from build123d import *

# Parameters (mm, degrees)
PAD004_DEPTH         = 30
SKETCH011_R          = 20.5
POCKET004_DEPTH      = 42.931486
POCKET004_DEPTH_BACK = 27.070514
POCKET005_DEPTH      = 263.838706
POCKET005_DEPTH_BACK = 247.977735
SKETCH013_R          = 2.7
POCKET006_DEPTH      = 220.90822
POCKET006_DEPTH_BACK = 250.90822
POCKET007_DEPTH      = 244.092718
SKETCH024_W          = 115.08152
SKETCH024_H          = 98.641312
POCKET017_DEPTH      = 2


with BuildPart() as part:
    # Sketch010 → Pad004 (new body)
    with BuildSketch(Plane.XZ):
        Polygon((-27.069514, 0), (-17.069514, 40), (32.930486, 40), (42.930486, 0), (32.930486, -40), (-17.069514, -40), align=None)
    extrude(amount=PAD004_DEPTH)

    # Sketch011 → Pocket004 (cut, two sides)
    with BuildSketch(Plane.YZ) as pocket004_sk:
        Circle(SKETCH011_R)
    extrude(amount=POCKET004_DEPTH, mode=Mode.SUBTRACT)
    extrude(pocket004_sk.sketch, amount=-POCKET004_DEPTH_BACK, mode=Mode.SUBTRACT)

    # Sketch012 → Pocket005 (cut, two sides)
    with BuildSketch(Plane.YZ) as pocket005_sk:
        Polygon((-36.13987, 42.447654), (-6.815503, 42.447654), (-6.815503, 35.734174), (-23.345354, 26.19066), (-36.13987, 13.396144), align=None)
    pocket005 = extrude(amount=POCKET005_DEPTH, mode=Mode.SUBTRACT) + extrude(pocket005_sk.sketch, amount=-POCKET005_DEPTH_BACK, mode=Mode.SUBTRACT)

    # Mirrored001: Pocket005 across Sketch012 H_Axis
    add(pocket005.mirror(Plane.XY), mode=Mode.SUBTRACT)

    # Sketch013 → Pocket006 (cut, two sides)
    with BuildSketch(Plane.XZ) as pocket006_sk:
        with Locations((-7.069514, 30)):
            Circle(SKETCH013_R)
        with Locations((22.930486, 30)):
            Circle(SKETCH013_R)
    pocket006 = extrude(amount=-POCKET006_DEPTH, mode=Mode.SUBTRACT) + extrude(pocket006_sk.sketch, amount=POCKET006_DEPTH_BACK, mode=Mode.SUBTRACT)

    # Mirrored002: Pocket006 across Sketch013 H_Axis
    add(pocket006.mirror(Plane(origin=(0, 0, 0), x_dir=(0, -1, 0), z_dir=(0, 0, 1))), mode=Mode.SUBTRACT)

    # Sketch014 (on Face5 of Mirrored002) → Pocket007 (cut, through all)
    with BuildSketch(Plane.XZ.offset(6.815503)):
        Polygon((-11.874352, 24.888732), (27.735323, 24.888732), (33.996942, 35.734174), (-18.135971, 35.734174), align=None)
    pocket007 = extrude(amount=POCKET007_DEPTH, mode=Mode.SUBTRACT)

    # Mirrored003: Pocket007 across Sketch014 H_Axis
    add(pocket007.mirror(Plane(origin=(0, -6.815503, 0), x_dir=(0, -1, 0), z_dir=(0, 0, 1))), mode=Mode.SUBTRACT)

    # Sketch024 (on Face12 of Mirrored003) → Pocket017 (cut)
    with BuildSketch(Plane(origin=(0, 0, 0), x_dir=(1, 0, 0), z_dir=(0, 1, 0))):
        with Locations((8.455631, -2.089874)):
            Rectangle(SKETCH024_W, SKETCH024_H)
    extrude(amount=-POCKET017_DEPTH, mode=Mode.SUBTRACT)


with BuildPart() as part_1:
    # Body003 placement: moved
    add(part.part.moved(Location((0, -40, 0))))


solid = part_1.part
Source: CAD feature listing. Evaluate the final solid. Frame: model axes, mm. A direction names the side the tool comes from. Give positions to 0.01 mm unless a question says otherwise; leave off trailing zeros. Loops run counter-clockwise (first coordinate to the right, second up) from the corner with the lowest first, then second, coordinate; pieces in that order, holes last. Notation, with made-up numbers: (-4, -31) -> (40, -31) arc R32 ccw to (40, -5) -> close; hole circle Ø11 at (9.5, 4). An arc over 180 degrees is marked (long way). Use a Markdown table: item, result. Add a question column.
1) Section query C-C, the plane x = -8.5. Return the cut outline in (y, z), then the cut area to 3 significant figures.
2) Line query: line 1 along Z through (x, y) = (-0.5, -44); line 2 along Z through (x, y) = (32, -50); line 3 along Z through (x, y) = (13.5, -61.5). Output: solid intervals per line, ascending. Write a range as [from, to].
3) Section query D-D, the plane x = 2. Return the cut outline in (y, z), then the cut area to 3 significant figures.
4) Section query A-A, the plane z = 31. Return the cut outline in (x, y).
5) First-contact query: pin 1 (5 mm diameter, centred on y = -67, z = -5, fed in from -X); pin 2 (8 mm diameter, centred on x = 4.5, z = -1, fed in from +Y); pin 3 (7.5 mm diameter, centred on x = 20, z = -31, fed in from -Y). Flat tips, straight axial feed; report the tip coordinate or a pass-through.
6) Pull-direction query (Z, two-part tool) for faces 1 (the face through (30.127, -53.625, -29.03)), 2 (the face through (-7.421, -44.441, -32.677)), 3 (the face through (37.86, -55.8, 20.28)); classes: +Z half, -Z half, draft (parallel to the pull), parting line (faces both ways), or undercut.
7) Reachability of faces 4 (the face through (-14.35, -53.63, 29.18)), 5 (the face through (8, -46.816, -33)), 6 (the face through (-17.396, -58.638, 28.908)) from +Z, -Z, +X, -X, +Y, -Y: full face, straight path, thin tool, end or side. Return the list, or none.
8) Section query B-B, the plane y = -44.25. Return the cut outline in (x, z), then the cut area to 3 significant figures.
Numbers:
| question | item | result |
|---|---|---|
| 1 | outline | (-70, -19.54) -> (-64.65, -24.89) -> (-46.82, -24.89) -> (-46.82, -27.71) -> (-42, -27.71) -> (-42, -20.4) arc R20.5 cw to (-42, 20.4) -> (-42, 27.71) -> (-46.82, 27.71) -> (-46.82, 24.89) -> (-64.65, 24.89) -> (-70, 19.54) -> close; (-46.82, -40) -> (-42, -40) -> (-42, -32.29) -> (-46.82, -32.29) -> close; (-46.82, 32.29) -> (-42, 32.29) -> (-42, 40) -> (-46.82, 40) -> close |
| 1 | area | 888 mm2 |
| 2 | line 1 | z = [-40, -20.11], [20.11, 40] |
| 2 | line 2 | z = [-32.28, -17.9], [17.9, 32.28] |
| 2 | line 3 | z = [-24.89, 24.89] |
| 3 | outline | (-70, -19.54) -> (-64.65, -24.89) -> (-46.82, -24.89) -> (-46.82, -40) -> (-42, -40) -> (-42, -20.4) arc R20.5 cw to (-42, 20.4) -> (-42, 40) -> (-46.82, 40) -> (-46.82, 24.89) -> (-64.65, 24.89) -> (-70, 19.54) -> close |
| 3 | area | 932 mm2 |
| 4 | outline | (-19.32, -55.02) -> (-15.4, -55.02) -> (-15.4, -46.82) -> (-9.58, -46.82) -> (-9.58, -42) -> (-19.32, -42) -> close; (-4.56, -46.82) -> (20.42, -46.82) -> (20.42, -42) -> (-4.56, -42) -> close; (25.44, -46.82) -> (31.26, -46.82) -> (31.26, -55.02) -> (35.18, -55.02) -> (35.18, -42) -> (25.44, -42) -> close |
| 5 | pin 1 | stops at x = -26.44 |
| 5 | pin 2 | stops at y = -59.88 |
| 5 | pin 3 | stops at y = -46.82 |
| 6 | face 1 | -Z half |
| 6 | face 2 | undercut |
| 6 | face 3 | +Z half |
| 7 | face 4 | +Z, -Y |
| 7 | face 5 | -Z, -Y |
| 7 | face 6 | +Z, +X, -X, -Y |
| 8 | outline | (-22.06, -20.05) -> (-17.07, -40) -> (32.93, -40) -> (37.92, -20.05) -> close; (-22.06, 20.05) -> (37.92, 20.05) -> (32.93, 40) -> (-17.07, 40) -> close; hole circle Ø5.4 at (-7.07, -30); hole circle Ø5.4 at (-7.07, 30); hole circle Ø5.4 at (22.93, -30); hole circle Ø5.4 at (22.93, 30) |
| 8 | area | 2,100 mm2 |
